Read the model definition and answer for the solid it produces. Units are mm, in the model's axes. Round coordinates to 2 decimals unless told otherwise and drop trailing zeros. Write each loop counter-clockwise with the first axis right and the second up, starting at its lowest first coordinate (ties: lowest second). Pieces come first, ordered by that corner, then holes. Notation, with made-up numbers: (-29.75, 61.25) - (17.25, 61.25) arc R30 cw to (17.25, 100.25) - close; hole circle Ø5 at (-32, 81.25). An arc over 180 degrees is marked (long way). Answer as CSV lines item,"result". Start each with the question number.
1) Find section C-C on x = -100. Determine the outline of the cut face in (y, z).
2) Find section D-D on y = -0.25. State how many separate pieces and enclosed holes the cut face has, then the cut area to 3 significant figures.
3) Consider line 1 along Z through (x, y) = (1, -0.5); line 2 along Z through (x, y) = (45, 10.5); line 3 along Z through (x, y) = (-112.5, 6.25). Determine where each line is inside the solid, lowest interval first.
4) Find section B-B on z = 76.5. Determine the outline of the cut face in (x, y).
5) Each of these flat-tipped pins is pushed along its axis until it touches: pin 1 (4 mm diameter, centred on x = 67, y = 0, fed in from +Z); pin 2 (4.5 mm diameter, centred on x = 100.5, y = 5.5, fed in from -Z); pin 3 (2 mm diameter, centred on y = 2.5, z = 18, fed in from +X). Where does it stop, or does it pass through?
6) Find section A-A on x = 0. Determine the outline of the cut face in (y, z), then the cut area to 3 significant figures.
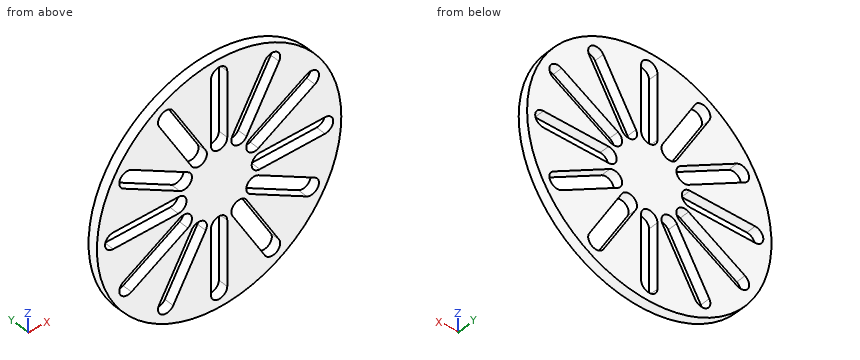
from build123d import *

# Parameters (mm, degrees)
SKETCH1_R           = 95.25
BOSS_EXTRUDE3_DEPTH = 7.62
SCALE1_SCALE        = 2


with BuildPart() as part:
    # Sketch1 → Boss-Extrude3 (new body)
    with BuildSketch(Plane(origin=(0, 0, 0), x_dir=(1, 0, 0), z_dir=(0, 1, 0))):
        Circle(SKETCH1_R)
        with BuildLine():
            Line((6.35, 82.55), (6.35, 31.75))
            ThreePointArc((6.35, 31.75), (0, 25.4), (-6.35, 31.75))
            Line((-6.35, 31.75), (-6.35, 82.55))
            ThreePointArc((-6.35, 82.55), (0, 88.9), (6.35, 82.55))
        make_face(mode=Mode.SUBTRACT)
        with BuildLine():
            Line((35.775738686, 74.665397082), (10.375738686, 30.67130657))
            ThreePointArc((10.375738686, 30.67130657), (12.7, 21.997045256), (21.374261314, 24.32130657))
            Line((21.374261314, 24.32130657), (46.774261314, 68.315397082))
            ThreePointArc((46.774261314, 68.315397082), (44.45, 76.989658396), (35.775738686, 74.665397082))
        make_face(mode=Mode.SUBTRACT)
        with BuildLine():
            Line((68.315397082, 46.774261314), (24.32130657, 21.374261314))
            ThreePointArc((24.32130657, 21.374261314), (21.997045256, 12.7), (30.67130657, 10.375738686))
            Line((30.67130657, 10.375738686), (74.665397082, 35.775738686))
            ThreePointArc((74.665397082, 35.775738686), (76.989658396, 44.45), (68.315397082, 46.774261314))
        make_face(mode=Mode.SUBTRACT)
        with BuildLine():
            Line((82.55, 6.35), (31.75, 6.35))
            ThreePointArc((31.75, 6.35), (25.4, 0), (31.75, -6.35))
            Line((31.75, -6.35), (82.55, -6.35))
            ThreePointArc((82.55, -6.35), (88.9, 0), (82.55, 6.35))
        make_face(mode=Mode.SUBTRACT)
        with BuildLine():
            Line((74.665397082, -35.775738686), (30.67130657, -10.375738686))
            ThreePointArc((30.67130657, -10.375738686), (21.997045256, -12.7), (24.32130657, -21.374261314))
            Line((24.32130657, -21.374261314), (68.315397082, -46.774261314))
            ThreePointArc((68.315397082, -46.774261314), (76.989658396, -44.45), (74.665397082, -35.775738686))
        make_face(mode=Mode.SUBTRACT)
        with BuildLine():
            Line((46.774261314, -68.315397082), (21.374261314, -24.32130657))
            ThreePointArc((21.374261314, -24.32130657), (12.7, -21.997045256), (10.375738686, -30.67130657))
            Line((10.375738686, -30.67130657), (35.775738686, -74.665397082))
            ThreePointArc((35.775738686, -74.665397082), (44.45, -76.989658396), (46.774261314, -68.315397082))
        make_face(mode=Mode.SUBTRACT)
        with BuildLine():
            Line((6.35, -82.55), (6.35, -31.75))
            ThreePointArc((6.35, -31.75), (0, -25.4), (-6.35, -31.75))
            Line((-6.35, -31.75), (-6.35, -82.55))
            ThreePointArc((-6.35, -82.55), (0, -88.9), (6.35, -82.55))
        make_face(mode=Mode.SUBTRACT)
        with BuildLine():
            Line((-35.775738686, -74.665397082), (-10.375738686, -30.67130657))
            ThreePointArc((-10.375738686, -30.67130657), (-12.7, -21.997045256), (-21.374261314, -24.32130657))
            Line((-21.374261314, -24.32130657), (-46.774261314, -68.315397082))
            ThreePointArc((-46.774261314, -68.315397082), (-44.45, -76.989658396), (-35.775738686, -74.665397082))
        make_face(mode=Mode.SUBTRACT)
        with BuildLine():
            Line((-68.315397082, -46.774261314), (-24.32130657, -21.374261314))
            ThreePointArc((-24.32130657, -21.374261314), (-21.997045256, -12.7), (-30.67130657, -10.375738686))
            Line((-30.67130657, -10.375738686), (-74.665397082, -35.775738686))
            ThreePointArc((-74.665397082, -35.775738686), (-76.989658396, -44.45), (-68.315397082, -46.774261314))
        make_face(mode=Mode.SUBTRACT)
        with BuildLine():
            Line((-82.55, -6.35), (-31.75, -6.35))
            ThreePointArc((-31.75, -6.35), (-25.4, 0), (-31.75, 6.35))
            Line((-31.75, 6.35), (-82.55, 6.35))
            ThreePointArc((-82.55, 6.35), (-88.9, 0), (-82.55, -6.35))
        make_face(mode=Mode.SUBTRACT)
        with BuildLine():
            Line((-74.665397082, 35.775738686), (-30.67130657, 10.375738686))
            ThreePointArc((-30.67130657, 10.375738686), (-21.997045256, 12.7), (-24.32130657, 21.374261314))
            Line((-24.32130657, 21.374261314), (-68.315397082, 46.774261314))
            ThreePointArc((-68.315397082, 46.774261314), (-76.989658396, 44.45), (-74.665397082, 35.775738686))
        make_face(mode=Mode.SUBTRACT)
        with BuildLine():
            Line((-46.774261314, 68.315397082), (-21.374261314, 24.32130657))
            ThreePointArc((-21.374261314, 24.32130657), (-12.7, 21.997045256), (-10.375738686, 30.67130657))
            Line((-10.375738686, 30.67130657), (-35.775738686, 74.665397082))
            ThreePointArc((-35.775738686, 74.665397082), (-44.45, 76.989658396), (-46.774261314, 68.315397082))
        make_face(mode=Mode.SUBTRACT)
    extrude(amount=BOSS_EXTRUDE3_DEPTH)


with BuildPart() as part_1:
    # Scale1: scaled about (0, 3.81, 0)
    add(part.part.scale(SCALE1_SCALE).moved(Location((0, -3.81, 0))))


solid = part_1.part
Check values:
1,outline,"(-3.81, -162.14) - (11.43, -162.14) - (11.43, -72.4) - (-3.81, -72.4) - close; (-3.81, -43.07) - (11.43, -43.07) - (11.43, -12.7) - (-3.81, -12.7) - close; (-3.81, 12.7) - (11.43, 12.7) - (11.43, 43.07) - (-3.81, 43.07) - close; (-3.81, 72.4) - (11.43, 72.4) - (11.43, 162.14) - (-3.81, 162.14) - close"
2,separate pieces,"1"
2,enclosed holes,"12"
2,area,"77,000 mm^2"
3,line 1,"z = -190.5 to -177.76, -50.84 to 50.84, 177.76 to 190.5"
3,line 2,"z = -185.11 to -103.34, -52.54 to -39.59, -23.91 to 23.91, 39.59 to 52.54, 103.34 to 185.11"
3,line 3,"z = -153.73 to -79.62, -50.29 to -12.7, 12.7 to 50.29, 79.62 to 153.73"
4,outline,"(-174.46, -3.81) - (-154.15, -3.81) - (-154.15, 11.43) - (-174.46, 11.43) - close; (-107.1, -3.81) - (-58.83, -3.81) - (-58.83, 11.43) - (-107.1, 11.43) - close; (-29.5, -3.81) - (-12.7, -3.81) - (-12.7, 11.43) - (-29.5, 11.43) - close; (12.7, -3.81) - (29.5, -3.81) - (29.5, 11.43) - (12.7, 11.43) - close; (58.83, -3.81) - (107.1, -3.81) - (107.1, 11.43) - (58.83, 11.43) - close; (154.15, -3.81) - (174.46, -3.81) - (174.46, 11.43) - (154.15, 11.43) - close"
5,pin 1,"stops at z = 179.07"
5,pin 2,"stops at z = -163.21"
5,pin 3,"stops at x = 189.74"
6,outline,"(-3.81, -190.5) - (11.43, -190.5) - (11.43, -177.8) - (-3.81, -177.8) - close; (-3.81, -50.8) - (11.43, -50.8) - (11.43, 50.8) - (-3.81, 50.8) - close; (-3.81, 177.8) - (11.43, 177.8) - (11.43, 190.5) - (-3.81, 190.5) - close"
6,area,"1,940 mm^2"
